Can you work these out from the model? Positions are in its coordinate system, mm. Face numbers are marked on the shaded views. Coordinates: 2 decimals unless noted, no trailing zeros. Order: outer loops, then holes, each group sorted by start corner. A loop starts at its lowest first (then second) coordinate and runs counter-clockwise, first axis right, second up. Notation, with made-up numbers: (31.25, 42) -> (78.25, 42) arc R26 ccw to (78.25, 61) -> close; hole circle Ø3 at (21, -8). An arc over 180 degrees is marked (long way). Use a Markdown table: item, result. Add a question column.
1. Suppose I cut it at D-D, the plane y = -37. List the corners of the cut face in (x, z) for me.
2. Suppose I cut it at A-A, the plane z = 53. List the corners of the cut face in (x, y) for me, then the cut area to 3 significant figures.
3. Suppose I cut it at C-C, the plane x = -35.5. List the corners of the cut face in (y, z) for me.
4. We'd pull the mould along X, two halves only. Please class the marked faces 1, 2 and 3: pulls with the +X half, pulls with the -X half, needs draft (parallel to the pull), parting line crosses it, or undercut.
5. Suppose I cut it at B-B, the plane y = 2.5. List the corners of the cut face in (x, z) for me, then the cut area to 3 significant figures.
6. For pin 1 Ø10 at (y, z) = (-17, 81.5) entering from +X; pin 2 Ø8 at (x, y) = (11.5, -32) entering from +Z; pin 3 Ø12 at (x, z) = (25.5, 78.5) entering from -Y, each with a flat end and sliding along its axis, tell me the tip position at first contact or that it passes through.
7. If I drill on line 1 along Y through (x, z) = (0, 64); line 2 along X through (y, z) = (0, -0.5); line 3 along Y through (x, z) = (-1, 49), over which ranges is the centre line in solid material (lowest first)? Write a range as from..to.
Solid Edge part; units mm, degrees
sketch "Sketch1" plane through (0, 0, 0) normal (0, 0, 1) x (1, 0, 0)
  circle A0 centre (0, 0) radius 25
  circle A1 centre (0, 0) radius 26.27
extrude "Protrusion1" add sketch "Sketch1" along normal blind 100
sketch "Sketch2" plane through (0, 0, 0) normal (0, 0, -1) x (1, 0, 0)
  circle A0 centre (0, 0) radius 55
extrude "ExtrudedProtrusion_2" add sketch "Sketch2" along normal blind 1.5875
sketch "Sketch3" plane through (0, 0, -1.5875) normal (0, 0, -1) x (0, 1, 0)
  circle A0 centre (0, 0) radius 0.127
extrude "Cutout1" cut sketch "Sketch3" against normal through all
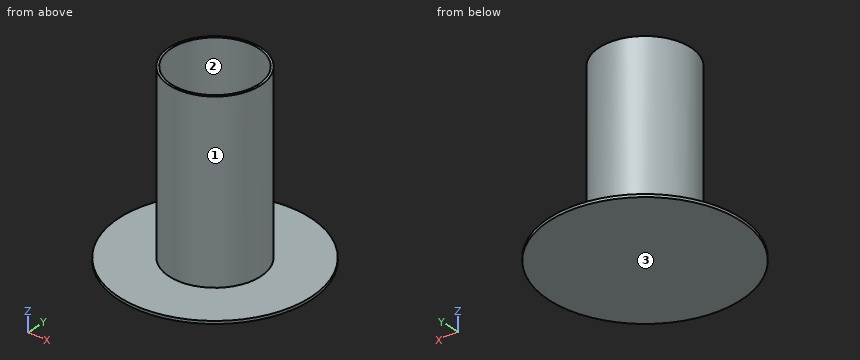
Worked out:
| question | item | result |
|---|---|---|
| 1 | outline | (-40.69, -1.59) -> (40.69, -1.59) -> (40.69, 0) -> (-40.69, 0) -> close |
| 2 | outline | circle Ø52.54 at (0, 0); hole circle Ø50 at (0, 0) |
| 2 | area | 205 mm² |
| 3 | outline | (-42.01, -1.59) -> (42.01, -1.59) -> (42.01, 0) -> (-42.01, 0) -> close |
| 4 | face 1 | parting line crosses it |
| 4 | face 2 | undercut |
| 4 | face 3 | needs draft |
| 5 | outline | (-54.94, -1.59) -> (54.94, -1.59) -> (54.94, 0) -> (26.15, 0) -> (26.15, 100) -> (24.87, 100) -> (24.87, 0) -> (-24.87, 0) -> (-24.87, 100) -> (-26.15, 100) -> (-26.15, 0) -> (-54.94, 0) -> close |
| 5 | area | 430 mm² |
| 6 | pin 1 | stops at x = 23.37 |
| 6 | pin 2 | stops at z = 0 |
| 6 | pin 3 | stops at y = -17.6 |
| 7 | line 1 | y = -26.27..-25, 25..26.27 |
| 7 | line 2 | x = -55..-0.13, 0.13..55 |
| 7 | line 3 | y = -26.25..-24.98, 24.98..26.25 |
